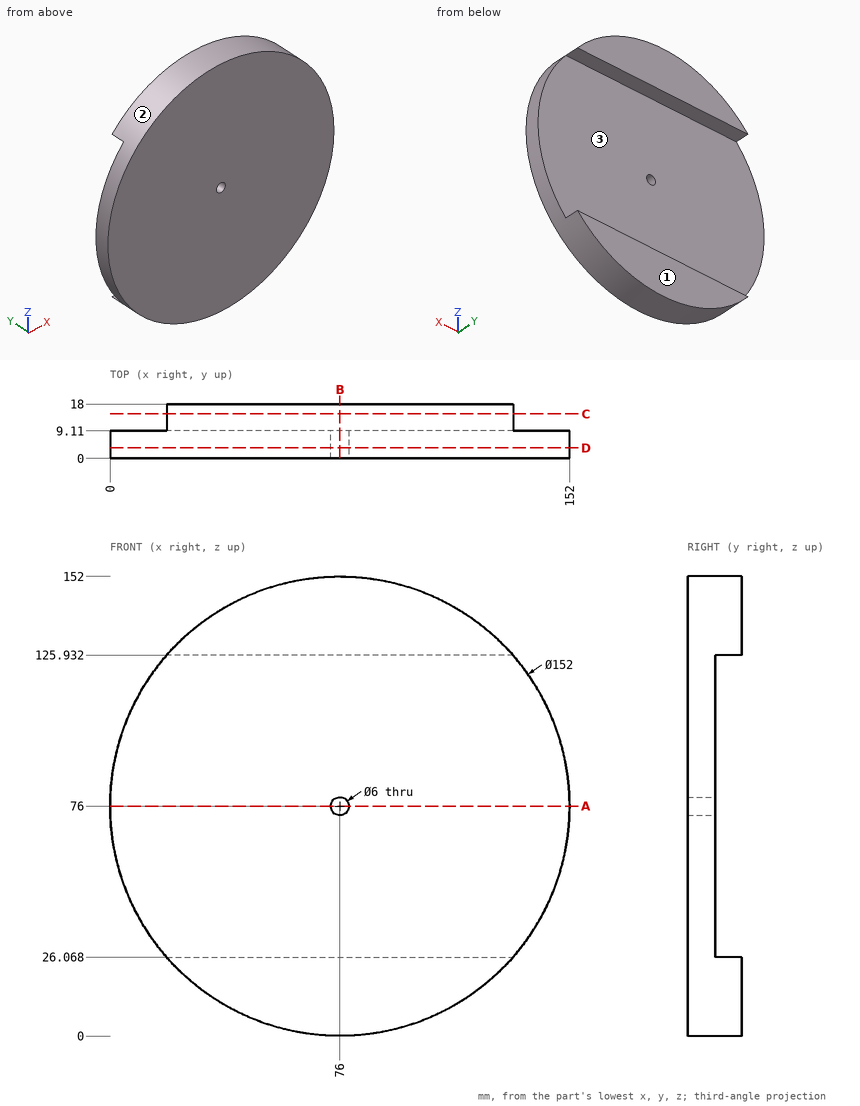
Can you work these out from the drawing? Everything is in mm from the part's minimum corner. Coordinates: 2 decimals unless noted, no trailing zeros. Loops run counter-clockwise (first coordinate to the right, second up) from the corner with the lowest first, then second, coordinate; pieces in that order, holes last. Notation, with made-up numbers: M -2,89 L 32,89 A17 ccw 32,117 Z; hole C -17,-12.75 d5. An arc over 180 degrees is marked long. Put each result on its own line as item: value. Start each with the question number.
(1) I need wall thicknesses on line 1 (X direction, y = 2, z = 76); line 2 (Z direction, x = 76, y = 11.75). Which ranges of each line are inside material? Lowest first, please. Write a range as from..to.
(2) Thinking about a two-plate mould opening in Z: for the marked faces 1, 2 and 3, which applies, pulls with the +Z half, pulls with the -Z half, needs draft (parallel to the pull), parting line crosses it, or undercut?
(3) Suppose I cut it at D-D on y = 3.5. Please give me the cut outline in (x, z), then the cut area to 3 significant figures.
(4) Suppose I cut it at C-C on y = 14.75. Please give me the cut outline in (x, z).
(5) Suppose I cut it at B-B on x = 76. Please give me the cut outline in (y, z).
(6) Will these pins go through, and if not, where does the flat tip stop? P1, Ø2, axis at y = 7.5, z = 31.5, coming from the +X side; P2, Ø6, axis at x = 78, z = 108.5, coming from the +Y side; P3, Ø4, axis at x = 54.5, y = 13.5, coming from the -Z side.
(7) Suppose I cut it at A-A on z = 76. Please give me the cut outline in (x, y), then the cut area to 3 significant figures.
Solutions:
1. line 1: x = 0..73, 79..152
1. line 2: z = 0..26.07, 125.93..152
2. face 1: needs draft
2. face 2: parting line crosses it
2. face 3: undercut
3. outline: C 76,76 d152; hole C 76,76 d6
3. area: 18,100 mm2
4. outline: M 18.7,26.07 A76 ccw 133.3,26.07 Z; M 18.7,125.93 L 133.3,125.93 A76 ccw Z
5. outline: M 0,0 L 18,0 L 18,26.07 L 9.11,26.07 L 9.11,73 L 0,73 Z; M 0,79 L 9.11,79 L 9.11,125.93 L 18,125.93 L 18,152 L 0,152 Z
6. P1: stops at x = 138.32
6. P2: stops at y = 9.11
6. P3: stops at z = 2.54
7. outline: M 0,0 L 73,0 L 73,9.11 L 0,9.11 Z; M 79,0 L 152,0 L 152,9.11 L 79,9.11 Z
7. area: 1,330 mm2
